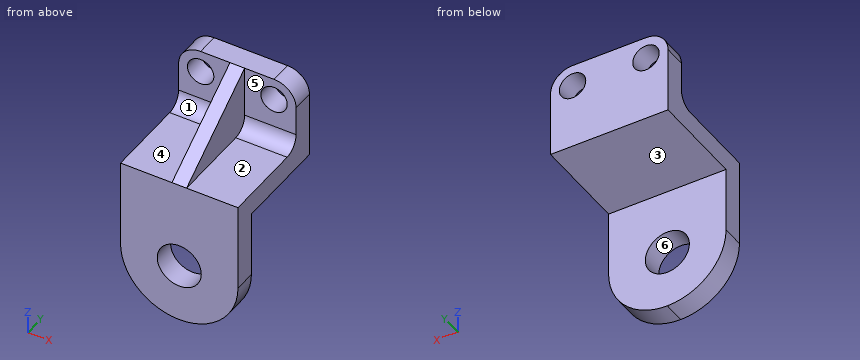
```python
from build123d import *

# Parameters (mm, degrees)
BOSS_EXTRUDE1_DEPTH     = 40
SKETCH2_W               = 15
SKETCH2_H               = 45
BOSS_EXTRUDE2_DEPTH     = 40
FILLET1_R               = 15
SKETCH9_R               = 9
CUT_EXTRUDE1_DEPTH      = 80
FILLET2_R               = 40
CUT_EXTRUDE6_DEPTH      = 171.367250374
CUT_EXTRUDE6_DEPTH_BACK = 171.367250374
SKETCH11_R              = 15
FILLET3_R               = 10
RIB17_REACH             = 172.367
SKETCH14_WALL_W         = 421.791442252
SKETCH14_WALL_H         = 10


with BuildPart() as part:
    # Sketch1 → Boss-Extrude1 (new, symmetric)
    with BuildSketch(Plane.YZ):
        Polygon((-65, 0), (-65, 85), (0, 85), (0, 100), (-80, 100), (-80, 0), align=None)
    extrude(amount=BOSS_EXTRUDE1_DEPTH, both=True)

    # Sketch2 → Boss-Extrude2 (add, symmetric)
    with BuildSketch(Plane.YZ):
        with Locations((-7.5, 122.5)):
            Rectangle(SKETCH2_W, SKETCH2_H)
    extrude(amount=BOSS_EXTRUDE2_DEPTH, both=True)

    # Fillet1
    fillet1_edges = [part.edges().sort_by_distance(p)[0] for p in [
        (-40, -7.5, 145),
        (40, -7.5, 145),
    ]]
    fillet(fillet1_edges, radius=FILLET1_R)

    # Sketch9 → Cut-Extrude1 (cut)
    with BuildSketch(Plane(origin=(0, 0, 0), x_dir=(-1, 0, 0), z_dir=(0, 1, 0))):
        with Locations(Location((25, 130, 0), (0, 0, 90))):
            Circle(SKETCH9_R)
        with Locations(Location((-25, 130, 0), (0, 0, 90))):
            Circle(SKETCH9_R)
    extrude(amount=-CUT_EXTRUDE1_DEPTH, mode=Mode.SUBTRACT)

    # Fillet2
    fillet2_edges = [part.edges().sort_by_distance(p)[0] for p in [
        (-40, -72.5, 0),
        (40, -72.5, 0),
    ]]
    fillet(fillet2_edges, radius=FILLET2_R - 0.0001)  # a hair under: the kernel refuses the full size

    # Sketch11 → Cut-Extrude6 (cut, two sides: drawn at the far end of the back side and taken through both)
    with BuildSketch(Plane.XZ.offset(80).offset(-CUT_EXTRUDE6_DEPTH_BACK)):
        with Locations(Location((0, 40, 0), (0, 0, 270))):
            Circle(SKETCH11_R)
    extrude(amount=CUT_EXTRUDE6_DEPTH + CUT_EXTRUDE6_DEPTH_BACK, mode=Mode.SUBTRACT)

    # Fillet3
    fillet3_edges = [part.edges().sort_by_distance(p)[0] for p in [
        (0, -15, 100),
    ]]
    fillet(fillet3_edges, radius=FILLET3_R)

    # Sketch14 wall → Rib17 (add, up to next)
    with BuildSketch(Plane(origin=(0, -47.5, 122.5), x_dir=(0, -0.822192191644, -0.56920997883), z_dir=(0, 0.56920997883, -0.822192191644)), mode=Mode.PRIVATE) as rib17_sk1:
        Rectangle(SKETCH14_WALL_W, SKETCH14_WALL_H)
    rib17_tool1 = extrude(rib17_sk1.sketch, amount=RIB17_REACH, mode=Mode.PRIVATE) - part.part
    add(rib17_tool1.solids().sort_by_distance((0, -47.5, 122.5))[0])


solid = part.part
```
Model file for the job. Use its own axes, mm. Face numbers are marked on the shaded views. A direction names the side the tool comes from. Round coordinates to 2 decimals unless told otherwise and drop trailing zeros. Loops run counter-clockwise (first coordinate to the right, second up) from the corner with the lowest first, then second, coordinate; pieces in that order, holes last. Notation, with made-up numbers: M 44.5,-30 L 72.5,-30 A21 cw 72.5,-7 Z; hole C 45.5,46.5 d9. An arc over 180 degrees is marked long. Put each result on its own line as item: value. Start each with the question number.
Item 1: Mould opens along Z. For the marked faces 4, 5 and 6 say: released by +Z, released by -Z, zero draft, split by the parting line, or undercut.
Item 2: Cut at B-B (x = -12.5). List the corners of the cut face in (y, z), then the cut area to 3 significant figures.
Item 3: Drop flat-ended pins along their axis: P1, Ø4, axis at x = 3, y = -20.5, coming from the +Z side; P2, Ø17.5, axis at x = 15.5, y = -53, coming from the +Z side; P3, Ø3, axis at x = -16.5, y = -65.5, coming from the -Z side. Give the stop position or say it passes through.
Item 4: Cut at D-D (z = 48). List the corners of the cut face in (x, y).
Item 5: Cut at C-C (y = -10.5). List the corners of the cut face in (x, z).
Item 6: Cut at A-A (y = -54). List the corners of the cut face in (x, z), then the cut area to 3 significant figures.
Item 7: 3-axis set-ups, long thin cutter, end or side, ignore diameter. For the marked faces 1, 2 and 3: which of +Z, -Z, +X, -X, +Y, -Y reach the whole face in a straight line?
Item 8: Drill centre lines: line 1 along X through (y, z) = (-4, 130); line 2 along X through (y, z) = (-69, 40); line 3 along Y through (x, z) = (5, 83). Where is each one in solid material? Low to high.
Answer block:
1. face 4: released by +Z
1. face 5: zero draft
1. face 6: undercut
2. outline: M -80,2 L -65,2 L -65,31.71 L -80,31.71 Z; M -80,48.29 L -65,48.29 L -65,85 L 0,85 L 0,145 L -15,145 L -15,110 A10 cw -25,100 L -80,100 Z
2. area: 2,890 mm2
3. P1: z = 142.58
3. P2: z = 100
3. P3: z = 2.92
4. outline: M -40,-80 L -12.69,-80 L -12.69,-65 L -40,-65 Z; M 12.69,-80 L 40,-80 L 40,-65 L 12.69,-65 Z
5. outline: M -40,85 L 40,85 L 40,130 A15 ccw 25,145 L -25,145 A15 ccw -40,130 Z; hole C -25,130 d18; hole C 25,130 d18
6. outline: M -40,85 L 40,85 L 40,100 L 5,100 L 5,118 L -5,118 L -5,100 L -40,100 Z
6. area: 1,380 mm2
7. face 1: +Z, -X, -Y
7. face 2: +Z, +X, -Y
7. face 3: -Z, +X, -X, +Y
8. line 1: -40 to -34, -16 to 16, 34 to 40
8. line 2: -40 to -15, 15 to 40
8. line 3: -80 to -65
